The drawing under review shows one solid part. Ordinate dimensions are in mm from its lowest x, y, z. A direction names the side the tool comes from. Round coordinates to 2 decimals unless told otherwise and drop trailing zeros. Write each loop counter-clockwise with the first axis right and the second up, starting at its lowest first coordinate (ties: lowest second). Pieces come first, ordered by that corner, then holes. Notation, with made-up numbers: (43, -25) -> (76, -25) arc R33 ccw to (76, 9) -> close; hole circle Ø11 at (44, 4). An arc over 180 degrees is marked (long way). Answer in a Markdown table with one row per item.
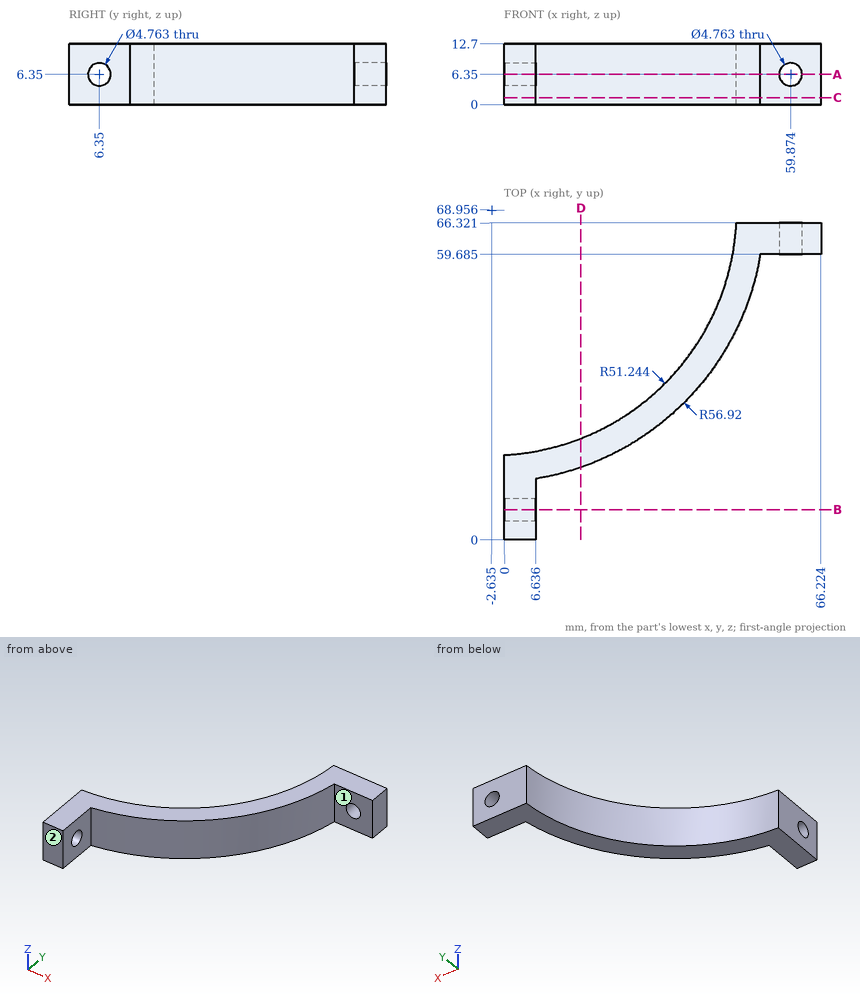
1) Consider section B-B on y = 6.35. State the section outline as (x, z) points (1 decimal).
Solved:
| item | result |
|---|---|
| outline | (0, 0) -> (6.6, 0) -> (6.6, 4) -> (0, 4) -> close; (0, 8.7) -> (6.6, 8.7) -> (6.6, 12.7) -> (0, 12.7) -> close |
2) For the marked faces 1 and 2, list the 3-axis set-ups (+Z, -Z, +X, -X, +Y, -Y) from which the entire face can be reached by the end or side of a thin tool; tool diameter is ignored.
Solved:
| item | result |
|---|---|
| face 1 | +Z, -Z, +X, -Y |
| face 2 | +Z, -Z, +X, -X, -Y |
3) Consider section A-A on z = 6.35. State the section outline as (x, y) points (1 decimal).
Solved:
| item | result |
|---|---|
| outline | (0, 0) -> (6.6, 0) -> (6.6, 4) -> (0, 4) -> close; (0, 8.7) -> (6.6, 8.7) -> (6.6, 12.8) arc R56.9 ccw to (53.5, 59.7) -> (57.5, 59.7) -> (57.5, 66.3) -> (48.5, 66.3) arc R51.2 cw to (0, 17.8) -> close; (62.3, 59.7) -> (66.2, 59.7) -> (66.2, 66.3) -> (62.3, 66.3) -> close |
4) Consider section D-D on x = 16. State the section outline as (y, z) points, then the cut area to 3 significant figures.
Solved:
| item | result |
|---|---|
| outline | (15.17, 0) -> (21.22, 0) -> (21.22, 12.7) -> (15.17, 12.7) -> close |
| area | 76.8 mm² |
5) Consider section C-C on z = 1.5. State the section outline as (x, y) points (1 decimal).
Solved:
| item | result |
|---|---|
| outline | (0, 0) -> (6.6, 0) -> (6.6, 12.8) arc R56.9 ccw to (53.5, 59.7) -> (66.2, 59.7) -> (66.2, 66.3) -> (48.5, 66.3) arc R51.2 cw to (0, 17.8) -> close |
6) For line 1 (X direction, y = 10.5, z = 3.25) (1 decimal); line 2 (Y direction, x = 56.5, z = 5) (1 decimal); line 3 (X direction, y = 37.5, z = 4.5) (1 decimal), list the stretches that pass through material, from the lowest coordinate up. Write a range as [from, to].
Solved:
| item | result |
|---|---|
| line 1 | [0, 6.6] |
| line 2 | [59.7, 66.3] |
| line 3 | [37.8, 44.8] |
7) Clearance check with flat-ended pins moving along their axes: pin 1 Ø6 at (x, z) = (22.5, 3) entering from -Y; pin 2 Ø1.5 at (y, z) = (29.5, 9) entering from -X (1 decimal); pin 3 Ø4 at (x, z) = (9, 2.5) entering from -Y. State where each tip first meets the part, or that it passes through.
Solved:
| item | result |
|---|---|
| pin 1 | y = 16.52 |
| pin 2 | x = 29.1 |
| pin 3 | y = 12.86 |
